from build123d import *

# Parameters (mm, degrees)
SKETCH_1_W                     = 50
SKETCH_1_H                     = 100
EXTRUDE_1_DEPTH                = 2
SKETCH_2_W                     = 3
SKETCH_2_H                     = 100
EXTRUDE_2_DEPTH                = 80
SKETCH_3_W                     = 2
SKETCH_3_H                     = 66.7
EXTRUDE_3_DEPTH                = 70
CUT_EXTRUDE_4_REACH            = 162.465
SKETCH_8_W                     = 2
SKETCH_8_H                     = 66.7
EXTRUDE_4_DEPTH                = 70
CUT_EXTRUDE_5_REACH            = 140.25
HOLE_WIZARD_M3_1_D             = 2.5
HOLE_WIZARD_M3_1_DEPTH         = 2
HOLE_WIZARD_M3_1_CSINK_D       = 3.05
HOLE_WIZARD_M3_1_CSINK_ANGLE   = 90
FILLET_1_R                     = 2
CUT_EXTRUDE_6_REACH            = 140.25
SKETCH_12_R                    = 11
CUT_EXTRUDE_7_REACH            = 162.465
SKETCH_13_R                    = 14.5
SKETCH_14_W                    = 2
SKETCH_14_H                    = 66.7
EXTRUDE_5_DEPTH                = 70
CUT_EXTRUDE_8_REACH            = 156.14
SKETCH_15_R                    = 5.1
CUT_EXTRUDE_9_DEPTH            = 155.140358116
CUT_EXTRUDE_9_DEPTH_BACK       = 155.140358116
SKETCH_19_W                    = 2
SKETCH_19_H                    = 66.7
CUT_EXTRUDE_10_DEPTH           = 119.844436134
FILLET_2_R                     = 2
HOLE_WIZARD_M3_3_D             = 2.5
HOLE_WIZARD_M3_3_CSINK_D       = 3.05
HOLE_WIZARD_M3_3_CSINK_ANGLE   = 90
CUT_EXTRUDE_11_DEPTH           = 134.88427839
CUT_EXTRUDE_11_DEPTH_BACK      = 134.88427839
SKETCH_28_W                    = 73
SKETCH_28_H                    = 100
HOLE_WIZARD_M2_5_1_D           = 2.05
HOLE_WIZARD_M2_5_1_CSINK_D     = 2.55
HOLE_WIZARD_M2_5_1_CSINK_ANGLE = 90


# Read off the part's stored shape, not the designer's step: M1.6 螺纹孔1, M1.6 螺纹孔2
with BuildPart() as part:
    # 草图1 → 凸台-拉伸1 (new body)
    with BuildSketch(Plane(origin=(0, 0, 0), x_dir=(1, 0, 0), z_dir=(0, 1, 0))):
        Rectangle(SKETCH_1_W, SKETCH_1_H)
    extrude(amount=EXTRUDE_1_DEPTH)

    # 草图2 → 凸台-拉伸2 (add)
    with BuildSketch(Plane(origin=(0, 2, 0), x_dir=(1, 0, 0), z_dir=(0, 1, 0))):
        with Locations((-23.5, 0)):
            Rectangle(SKETCH_2_W, SKETCH_2_H)
    extrude(amount=EXTRUDE_2_DEPTH)

    # 草图3 → 凸台-拉伸3 (add)
    with BuildSketch(Plane.ZY.offset(25)):
        with Locations((-49, 48.65)):
            Rectangle(SKETCH_3_W, SKETCH_3_H)
    extrude(amount=EXTRUDE_3_DEPTH)

    # 草图4 → 切除-拉伸4 (cut, up to next)
    with BuildSketch(Plane(origin=(0, 0, -50), x_dir=(-1, 0, 0), z_dir=(0, 0, -1)), mode=Mode.PRIVATE) as cut_extrude_4_sk1:
        with BuildLine():
            Line((95, 82), (61.65, 82))
            ThreePointArc((61.65, 82), (85.232011153, 72.232011153), (95, 48.65))
            Line((95, 48.65), (95, 82))
        make_face()
    cut_extrude_4_tool1 = extrude(cut_extrude_4_sk1.sketch, amount=-CUT_EXTRUDE_4_REACH, mode=Mode.PRIVATE) & part.part
    # 草图4 → 切除-拉伸4 (cut, up to next)
    with BuildSketch(Plane(origin=(0, 0, -50), x_dir=(-1, 0, 0), z_dir=(0, 0, -1)), mode=Mode.PRIVATE) as cut_extrude_4_sk2:
        with BuildLine():
            ThreePointArc((95, 48.65), (85.232011153, 25.067988847), (61.65, 15.3))
            Line((61.65, 15.3), (95, 15.3))
            Line((95, 15.3), (95, 48.65))
        make_face()
    cut_extrude_4_tool2 = extrude(cut_extrude_4_sk2.sketch, amount=-CUT_EXTRUDE_4_REACH, mode=Mode.PRIVATE) & part.part
    add(cut_extrude_4_tool1.solids().sort_by_distance((-87.550679, 74.550679, -50))[0], mode=Mode.SUBTRACT)
    add(cut_extrude_4_tool2.solids().sort_by_distance((-87.550679, 22.749321, -50))[0], mode=Mode.SUBTRACT)

    # 草图8 → 凸台-拉伸4 (add)
    with BuildSketch(Plane.ZY.offset(25)):
        with Locations((7, 48.65)):
            Rectangle(SKETCH_8_W, SKETCH_8_H)
    extrude(amount=EXTRUDE_4_DEPTH)

    # 草图9 → 切除-拉伸5 (cut, up to next)
    with BuildSketch(Plane.XY.offset(8), mode=Mode.PRIVATE) as cut_extrude_5_sk1:
        with BuildLine():
            ThreePointArc((-95, 48.65), (-85.232011153, 72.232011153), (-61.65, 82))
            Line((-61.65, 82), (-95, 82))
            Line((-95, 82), (-95, 48.65))
        make_face()
    cut_extrude_5_tool1 = extrude(cut_extrude_5_sk1.sketch, amount=-CUT_EXTRUDE_5_REACH, mode=Mode.PRIVATE) & part.part
    # 草图9 → 切除-拉伸5 (cut, up to next)
    with BuildSketch(Plane.XY.offset(8), mode=Mode.PRIVATE) as cut_extrude_5_sk2:
        with BuildLine():
            ThreePointArc((-61.65, 15.3), (-85.232011153, 25.067988847), (-95, 48.65))
            Line((-95, 48.65), (-95, 15.3))
            Line((-95, 15.3), (-61.65, 15.3))
        make_face()
    cut_extrude_5_tool2 = extrude(cut_extrude_5_sk2.sketch, amount=-CUT_EXTRUDE_5_REACH, mode=Mode.PRIVATE) & part.part
    add(cut_extrude_5_tool1.solids().sort_by_distance((-87.550679, 74.550679, 8))[0], mode=Mode.SUBTRACT)
    add(cut_extrude_5_tool2.solids().sort_by_distance((-87.550679, 22.749321, 8))[0], mode=Mode.SUBTRACT)

    # M3 螺纹孔1
    with Locations(Plane.XY.offset(8)):
        with Locations((-78.970508076, 38.65), (-61.65, 68.65), (-44.329491924, 38.65)):
            CounterSinkHole(HOLE_WIZARD_M3_1_D / 2, HOLE_WIZARD_M3_1_CSINK_D / 2, depth=HOLE_WIZARD_M3_1_DEPTH, counter_sink_angle=HOLE_WIZARD_M3_1_CSINK_ANGLE)

    # 圆角1
    fillet_1_edges = [part.edges().sort_by_distance(p)[0] for p in [
        (-23.5, 82, 50),
        (25, 1, 50),
        (25, 1, -50),
    ]]
    fillet(fillet_1_edges, radius=FILLET_1_R)

    # 草图12 → 切除-拉伸6 (cut, up to next)
    with BuildSketch(Plane.XY.offset(8), mode=Mode.PRIVATE) as cut_extrude_6_sk1:
        with Locations((-61.65, 48.65)):
            Circle(SKETCH_12_R)
    cut_extrude_6_tool1 = extrude(cut_extrude_6_sk1.sketch, amount=-CUT_EXTRUDE_6_REACH, mode=Mode.PRIVATE) & part.part
    add(cut_extrude_6_tool1.solids().sort_by_distance((-61.65, 48.65, 8))[0], mode=Mode.SUBTRACT)

    # 草图13 → 切除-拉伸7 (cut, up to next)
    with BuildSketch(Plane(origin=(0, 0, -50), x_dir=(-1, 0, 0), z_dir=(0, 0, -1)), mode=Mode.PRIVATE) as cut_extrude_7_sk1:
        with Locations((61.65, 48.65)):
            Circle(SKETCH_13_R)
    cut_extrude_7_tool1 = extrude(cut_extrude_7_sk1.sketch, amount=-CUT_EXTRUDE_7_REACH, mode=Mode.PRIVATE) & part.part
    add(cut_extrude_7_tool1.solids().sort_by_distance((-61.65, 48.65, -50))[0], mode=Mode.SUBTRACT)

    # 草图14 → 凸台-拉伸5 (add)
    with BuildSketch(Plane.ZY.offset(25)):
        with Locations((-38.5, 48.65)):
            Rectangle(SKETCH_14_W, SKETCH_14_H)
    extrude(amount=EXTRUDE_5_DEPTH)

    # 草图15 → 切除-拉伸8 (cut, up to next)
    with BuildSketch(Plane(origin=(0, 0, -39.5), x_dir=(-1, 0, 0), z_dir=(0, 0, -1)), mode=Mode.PRIVATE) as cut_extrude_8_sk1:
        with Locations(Location((61.65, 48.65, 0), (0, 0, 90))):
            Circle(SKETCH_15_R)
    cut_extrude_8_tool1 = extrude(cut_extrude_8_sk1.sketch, amount=-CUT_EXTRUDE_8_REACH, mode=Mode.PRIVATE) & part.part
    add(cut_extrude_8_tool1.solids().sort_by_distance((-61.65, 48.65, -39.5))[0], mode=Mode.SUBTRACT)

    # 草图18 → 切除-拉伸9 (cut, two sides: drawn at the far end of the back side and taken through both)
    with BuildSketch(Plane(origin=(0, 0, -39.5), x_dir=(-1, 0, 0), z_dir=(0, 0, -1)).offset(-CUT_EXTRUDE_9_DEPTH_BACK)):
        with BuildLine():
            Line((95, 15.3), (95, 48.65))
            ThreePointArc((95, 48.65), (85.232011153, 25.067988847), (61.65, 15.3))
            Line((61.65, 15.3), (95, 15.3))
        make_face()
        with BuildLine():
            Line((95, 48.65), (95, 82))
            Line((95, 82), (61.65, 82))
            ThreePointArc((61.65, 82), (85.232011153, 72.232011153), (95, 48.65))
        make_face()
    extrude(amount=CUT_EXTRUDE_9_DEPTH + CUT_EXTRUDE_9_DEPTH_BACK, mode=Mode.SUBTRACT)

    # 草图19 → 切除-拉伸10 (cut, through all)
    with BuildSketch(Plane.ZY.offset(25)):
        with Locations((-49, 48.65)):
            Rectangle(SKETCH_19_W, SKETCH_19_H)
    extrude(amount=CUT_EXTRUDE_10_DEPTH, mode=Mode.SUBTRACT)

    # 圆角2
    fillet_2_edges = [part.edges().sort_by_distance(p)[0] for p in [
        (-23.5, 82, -50),
    ]]
    fillet(fillet_2_edges, radius=FILLET_2_R)

    # M3 螺纹孔3 (through all)
    with Locations(Plane(origin=(0, 2, 0), x_dir=(1, 0, 0), z_dir=(0, 1, 0))):
        with Locations((-2.7, 0), (21, 10), (21, -10)):
            CounterSinkHole(HOLE_WIZARD_M3_3_D / 2, HOLE_WIZARD_M3_3_CSINK_D / 2, counter_sink_angle=HOLE_WIZARD_M3_3_CSINK_ANGLE)

    # M1.6 螺纹孔1 outline → M1.6 螺纹孔1 (revolve, cut)
    with BuildSketch(Plane(origin=(10, 0, -28), x_dir=(1, 0, 0), z_dir=(0, 0, 1))):
        Polygon((0, 0), (0.625, 0), (0.625, 1.8), (0.825, 2), (0, 2), align=None)
    revolve(axis=Axis((10, 0, -28), (0, 1, 0)), mode=Mode.SUBTRACT)

    # Hole Wizard M1.6 _1 2 outline → Hole Wizard M1.6 _1 2 (revolve, cut)
    with BuildSketch(Plane(origin=(6.4, 0, -28), x_dir=(1, 0, 0), z_dir=(0, 0, 1))):
        Polygon((0, 0), (0.625, 0), (0.625, 1.8), (0.825, 2), (0, 2), align=None)
    revolve(axis=Axis((6.4, 0, -28), (0, 1, 0)), mode=Mode.SUBTRACT)

    # M1.6 螺纹孔2 outline → M1.6 螺纹孔2 (revolve, cut)
    with BuildSketch(Plane(origin=(10, 0, -22), x_dir=(1, 0, 0), z_dir=(0, 0, 1))):
        Polygon((0, 0), (0.625, 0), (0.625, 1.8), (0.825, 2), (0, 2), align=None)
    revolve(axis=Axis((10, 0, -22), (0, 1, 0)), mode=Mode.SUBTRACT)

    # Hole Wizard M1.6 _2 2 outline → Hole Wizard M1.6 _2 2 (revolve, cut)
    with BuildSketch(Plane(origin=(6.4, 0, -22), x_dir=(1, 0, 0), z_dir=(0, 0, 1))):
        Polygon((0, 0), (0.625, 0), (0.625, 1.8), (0.825, 2), (0, 2), align=None)
    revolve(axis=Axis((6.4, 0, -22), (0, 1, 0)), mode=Mode.SUBTRACT)

    # 草图28 → 切除-拉伸11 (cut, two sides: drawn at the far end of the back side and taken through both)
    with BuildSketch(Plane(origin=(0, 2, 0), x_dir=(1, 0, 0), z_dir=(0, 1, 0)).offset(-CUT_EXTRUDE_11_DEPTH_BACK)):
        with Locations((-58.5, 0)):
            Rectangle(SKETCH_28_W, SKETCH_28_H)
    extrude(amount=CUT_EXTRUDE_11_DEPTH + CUT_EXTRUDE_11_DEPTH_BACK, mode=Mode.SUBTRACT)

    # M2.5 螺纹孔1 (through all)
    with Locations(Plane(origin=(0, 2, 0), x_dir=(1, 0, 0), z_dir=(0, 1, 0))):
        with Locations((-18, 4), (-18, -4)):
            CounterSinkHole(HOLE_WIZARD_M2_5_1_D / 2, HOLE_WIZARD_M2_5_1_CSINK_D / 2, counter_sink_angle=HOLE_WIZARD_M2_5_1_CSINK_ANGLE)


solid = part.part
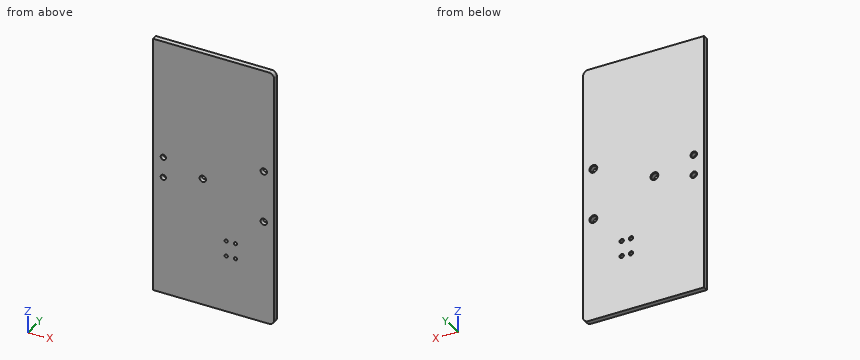
Read the model definition and answer for the solid it produces. Units are mm, in the model's axes. Round coordinates to 2 decimals unless told otherwise and drop trailing zeros. Loops run counter-clockwise (first coordinate to the right, second up) from the corner with the lowest first, then second, coordinate; pieces in that order, holes last.
Q1. Section B-B on x = -18 is taken. Write down the section's boundary in (y, z) (3 decimals), and give its area (3 significant figures).
Q2. Section A-A on z = 4 is taken. Write down the section's boundary in (x, y) (3 decimals), and give its area (3 significant figures).
Q3. This flat-tipped pin is pushed along its axis until it touches: pin 1 (1.4 mm diameter, centred on x = 6.4, z = -22, fed in from -Y). Where does it stop, or does it pass through?
Q4. Consider probe 1 along Z at (x, y) = (21, 0.7); probe 2 along Z at (x, y) = (-18, 1.2) (3 decimals); probe 3 along X at (y, z) = (0.75, -10). Determine where each line is inside the solid, lowest interval first.
Output:
1. outline: (0, -50) - (2, -50) - (2, -5.275) - (1.75, -5.025) - (0, -5.025) - close; (0, -2.975) - (1.75, -2.975) - (2, -2.725) - (2, 2.725) - (1.75, 2.975) - (0, 2.975) - close; (0, 5.025) - (1.75, 5.025) - (2, 5.275) - (2, 50) - (0, 50) - close
1. area: 192 mm2
2. outline: (-22, 0) - (-19.025, 0) - (-19.025, 1.75) - (-19.275, 2) - (-22, 2) - close; (-16.975, 0) - (25, 0) - (25, 2) - (-16.725, 2) - (-16.975, 1.75) - close
2. area: 89.8 mm2
3. pin 1: stops at y = 0
4. probe 1: z = -50 to -11.25, -8.75 to 8.75, 11.25 to 50
4. probe 2: z = -50 to -5.025, -2.975 to 2.975, 5.025 to 50
4. probe 3: x = -22 to 19.75, 22.25 to 25
